Here's the drawing with two shaded views (mm, measured from the low corner). I have some questions. Coordinates: 2 decimals unless noted, no trailing zeros. Loops run counter-clockwise (first coordinate to the right, second up) from the corner with the lowest first, then second, coordinate; pieces in that order, holes last.
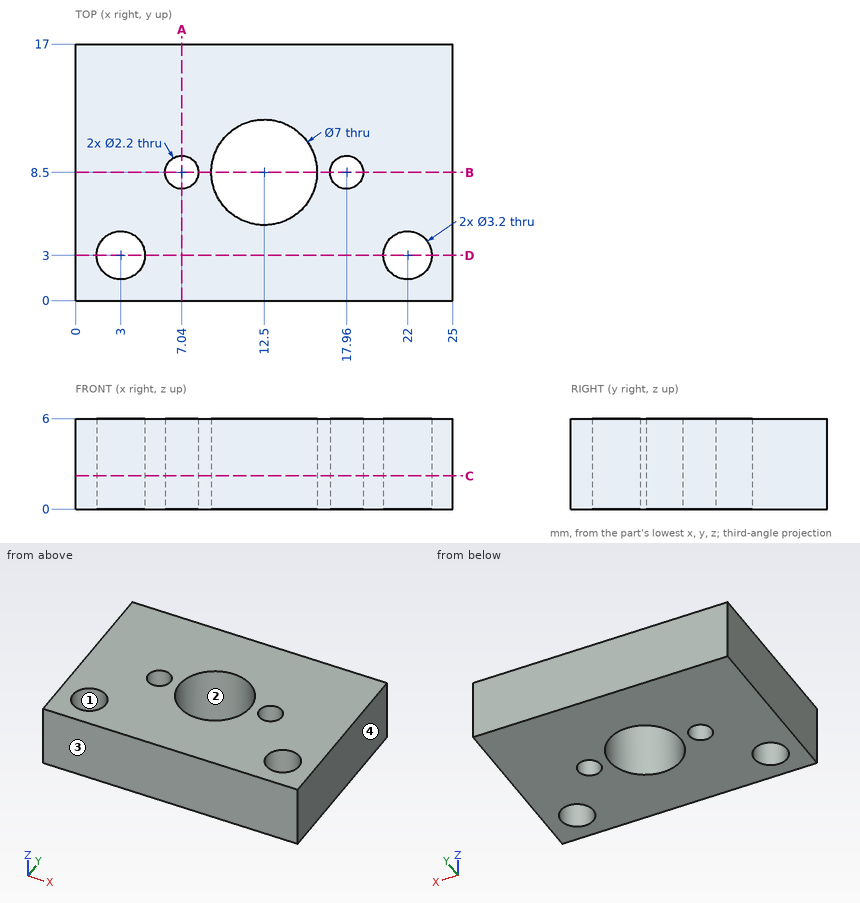
(1) I want a section at D-D on y = 3. Write out the boundary of the cut face in (x, z), then the cut area to 3 significant figures.
Check values:
outline: (0, 0) - (1.4, 0) - (1.4, 6) - (0, 6) - close; (4.6, 0) - (20.4, 0) - (20.4, 6) - (4.6, 6) - close; (23.6, 0) - (25, 0) - (25, 6) - (23.6, 6) - close
area: 112 mm2
(2) If we mould it in two halves opening along Y, with no side actions, what happens to the marked faces 1, 2, 3 and 4? For each: released by +Y, released by -Y, zero draft, split by the parting line, or undercut.
Check values:
face 1: undercut
face 2: undercut
face 3: released by -Y
face 4: zero draft
(3) I want a section at C-C on z = 2.2. Write out the boundary of the cut face in (x, y), then the cut area to 3 significant figures.
Check values:
outline: (0, 0) - (25, 0) - (25, 17) - (0, 17) - close; hole circle Ø3.2 at (3, 3); hole circle Ø2.2 at (7.04, 8.5); hole circle Ø7 at (12.5, 8.5); hole circle Ø2.2 at (17.96, 8.5); hole circle Ø3.2 at (22, 3)
area: 363 mm2
(4) I want a section at A-A on x = 7.04. Write out the boundary of the cut face in (y, z), then the cut area to 3 significant figures.
Check values:
outline: (0, 0) - (7.4, 0) - (7.4, 6) - (0, 6) - close; (9.6, 0) - (17, 0) - (17, 6) - (9.6, 6) - close
area: 88.8 mm2
(5) I want a section at B-B on y = 8.5. Write out the boundary of the cut face in (x, z), then the cut area to 3 significant figures.
Check values:
outline: (0, 0) - (5.94, 0) - (5.94, 6) - (0, 6) - close; (8.14, 0) - (9, 0) - (9, 6) - (8.14, 6) - close; (16, 0) - (16.86, 0) - (16.86, 6) - (16, 6) - close; (19.06, 0) - (25, 0) - (25, 6) - (19.06, 6) - close
area: 81.6 mm2
(6) If I drill on probe 1 along Y at (x, z) = (22, 4.45); probe 2 along Y at (x, z) = (12.5, 4.35); probe 3 along X at (y, z) = (6.5, 3.45), over which ranges is the centre line in solid material (lowest first)?
Check values:
probe 1: y = 0 to 1.4, 4.6 to 17
probe 2: y = 0 to 5, 12 to 17
probe 3: x = 0 to 9.63, 15.37 to 25
